Check sheet for the drawn part. Datum: minimum x, y, z corner. Units: mm. A direction names the side the tool comes from. Give positions to 0.01 mm unless a question says otherwise; leave off trailing zeros. Order: outer loops, then holes, each group sorted by start corner. A loop starts at its lowest first (then second) coordinate and runs counter-clockwise, first axis right, second up. Notation, with made-up numbers: M -31,46.5 L 11,46.5 A26 ccw 11,72.5 Z; hole C 31,63.25 d8. An arc over 180 degrees is marked long. Answer in a Markdown table with one row per item. Add a question column.
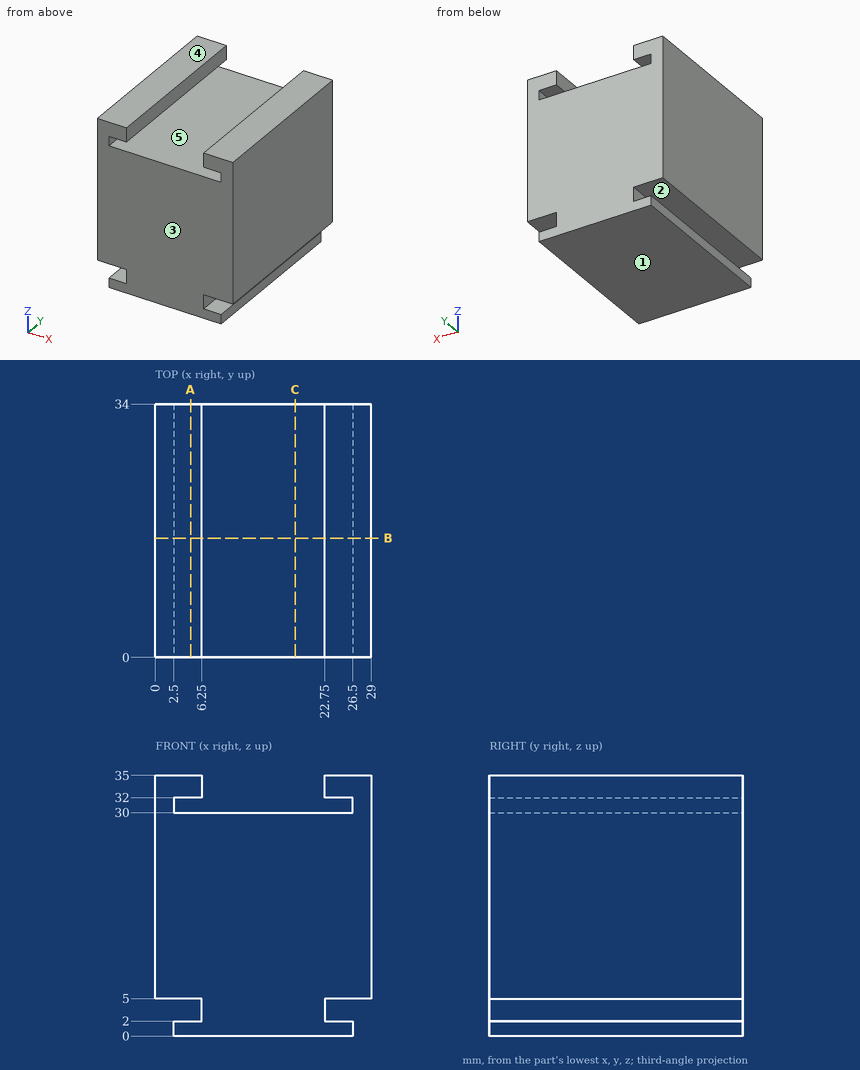
Q1. Go/stop test with flat-tipped pins: pin 1 (1.6 mm diameter, centred on y = 21.5, z = 1.5, fed in from +X); pin 2 (3 mm diameter, centred on x = 2, y = 19, fed in from -Z); pin 3 (2.5 mm diameter, centred on y = 12.5, z = 3.5, fed in from +X); pin 4 (1 mm diameter, centred on y = 10, z = 1.5, fed in from -X). Record where each tip stops, or that it passes through.
Q2. Cross-section at A-A (x = 4.75). Record the boundary of the cut face in (y, z).
Q3. Draft check along Z on the marked faces 3, 4 and 5. Enter one of: pulls with the +Z half, pulls with the -Z half, needs draft (parallel to the pull), parting line crosses it, or undercut.
Q4. Tool access check on the marked faces 1 and 2. Record the directions out of +Z, -Z, +X, -X, +Y, -Y that give a thin tool (end or side, any length) a straight path to the whole face; none if there is none.
Q5. Thickness scan on probe 1 along Z at (x, y) = (25.25, 23); probe 2 along X at (y, z) = (9, 31); probe 3 along Z at (x, y) = (27, 13.5). Record the ranges inside material, lowest first.
Q6. Cross-section at B-B (y = 16). Record the boundary of the cut face in (x, z).
Q7. Cross-section at C-C (x = 18.75). Record the boundary of the cut face in (y, z), and give its area (3 significant figures).
Values follow:
| question | item | result |
|---|---|---|
| 1 | pin 1 | x = 26.5 |
| 1 | pin 2 | z = 0 |
| 1 | pin 3 | x = 22.75 |
| 1 | pin 4 | x = 2.5 |
| 2 | outline | M 0,0 L 34,0 L 34,2 L 0,2 Z; M 0,5 L 34,5 L 34,30 L 0,30 Z; M 0,32 L 34,32 L 34,35 L 0,35 Z |
| 3 | face 3 | needs draft |
| 3 | face 4 | pulls with the +Z half |
| 3 | face 5 | undercut |
| 4 | face 1 | -Z, +X, -X, +Y, -Y |
| 4 | face 2 | -X, +Y, -Y |
| 5 | probe 1 | 0 to 2, 5 to 30, 32 to 35 |
| 5 | probe 2 | 0 to 2.5, 26.5 to 29 |
| 5 | probe 3 | 5 to 35 |
| 6 | outline | M 0,5 L 6.25,5 L 6.25,2 L 2.5,2 L 2.5,0 L 26.5,0 L 26.5,2 L 22.75,2 L 22.75,5 L 29,5 L 29,35 L 22.75,35 L 22.75,32 L 26.5,32 L 26.5,30 L 2.5,30 L 2.5,32 L 6.25,32 L 6.25,35 L 0,35 Z |
| 7 | outline | M 0,0 L 34,0 L 34,30 L 0,30 Z |
| 7 | area | 1,020 mm² |
